Read the model definition and answer for the solid it produces. Units are mm, in the model's axes. Coordinates: 2 decimals unless noted, no trailing zeros. Write each loop counter-clockwise with the first axis right and the second up, starting at its lowest first coordinate (ties: lowest second). Pieces come first, ordered by that corner, then holes. Notation, with made-up numbers: (24.5, 86) -> (48.5, 86) arc R14 ccw to (48.5, 110) -> close; hole circle Ø8 at (4.5, 43). An arc over 180 degrees is marked (long way). Answer in a Markdown table with one row per item. Add a question column.
Item 1: Section C-C on y = 2.4 is taken. Count the separate pieces of the cut face and the enclosed holes in it, then the cut area to 3 significant figures.
Item 2: Given pin 1 Ø0.9 at (x, y) = (148, 2) entering from -Z; pin 2 Ø0.9 at (y, z) = (1, -73.5) entering from -X, each flat-ended and moving along its own axis, determine where each tip first touches the part or whether it passes through.
Item 3: Section A-A on z = -174 is taken. Write down the section's boundary in (x, y), then the cut area to 3 significant figures.
Item 4: Section B-B on z = -23 is taken. Write down the section's boundary in (x, y), then the cut area to 3 significant figures.
Item 5: Straight lines are drawn through the part: line 1 (X direction, y = 1.9, z = -97); line 2 (X direction, y = 1.95, z = -175.5); line 3 (Z direction, x = 139.2, y = 2). For each, find the intervals that lie inside material, in ascending order. Write a range as from..to.
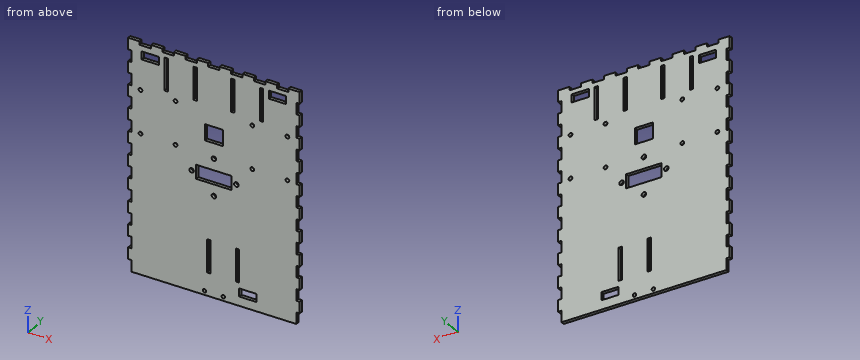
```python
from build123d import *

# Parameters (mm, degrees)
MDFESB_W          = 150
MDFESB_H          = 200
MDF_DEPTH         = 3
LDRESB_W          = 3
LDRESB_H          = 28.5
LDRESB_W_2        = 15
LDRESB_H_2        = 7
LDRBURACOS_DEPTH  = 3
CORESB_R          = 2
CORESB_W          = 31.12
CORESB_H          = 12.13
CORBURACOS_DEPTH  = 3
ENCAIXESESB_W     = 10
ENCAIXESESB_H     = 3
ENCAIXESESB_W_2   = 3
ENCAIXESESB_H_2   = 10
ENCAIXE_DEPTH     = 3
ACOPLMOTORESB_R   = 1.65
ACOPLMOTORESB_W   = 16
ACOPLMOTORESB_H   = 14
ACOPLMOTOR_DEPTH  = 3
CASTERFUROSESB_R  = 1.5
CASTERFUROS_DEPTH = 3


with BuildPart() as part:
    # mdfEsb → mdf (new body)
    with BuildSketch(Plane(origin=(0, 0, 0), x_dir=(1, 0, 0), z_dir=(0, 1, 0))):
        with Locations((75, 100)):
            Rectangle(MDFESB_W, MDFESB_H)
    extrude(amount=MDF_DEPTH)

    # ldrEsb → ldrBuracos (cut)
    with BuildSketch(Plane(origin=(0, 3, 0), x_dir=(1, 0, 0), z_dir=(0, 1, 0))):
        with Locations((33.4, 21.25)):
            Rectangle(LDRESB_W, LDRESB_H)
        with Locations((58.5, 21.25)):
            Rectangle(LDRESB_W, LDRESB_H)
        with Locations((91.5, 21.25)):
            Rectangle(LDRESB_W, LDRESB_H)
        with Locations((116.6, 21.25)):
            Rectangle(LDRESB_W, LDRESB_H)
        with Locations((70.5, 165.75)):
            Rectangle(LDRESB_W, LDRESB_H)
        with Locations((95.6, 165.75)):
            Rectangle(LDRESB_W, LDRESB_H)
        with Locations((130.6, 10.5)):
            Rectangle(LDRESB_W_2, LDRESB_H_2)
        with Locations((19.4, 11.5)):
            Rectangle(LDRESB_W_2, LDRESB_H_2)
        with Locations((104.6, 188.5)):
            Rectangle(LDRESB_W_2, LDRESB_H_2)
    extrude(amount=-LDRBURACOS_DEPTH, mode=Mode.SUBTRACT)

    # corEsb → corBuracos (cut)
    with BuildSketch(Plane(origin=(0, 3, 0), x_dir=(1, 0, 0), z_dir=(0, 1, 0))):
        with Locations(Location((75, 112.63, 0), (0, 0, 270))):
            Circle(CORESB_R)
        with Locations(Location((75, 80.5, 0), (0, 0, 270))):
            Circle(CORESB_R)
        with Locations(Location((94.56, 96.565, 0), (0, 0, 270))):
            Circle(CORESB_R)
        with Locations(Location((55.44, 96.565, 0), (0, 0, 270))):
            Circle(CORESB_R)
        with Locations((75, 96.565)):
            Rectangle(CORESB_W, CORESB_H)
    extrude(amount=-CORBURACOS_DEPTH, mode=Mode.SUBTRACT)

    # EncaixesEsb → Encaixe (cut)
    with BuildSketch(Plane(origin=(0, 3, 0), x_dir=(1, 0, 0), z_dir=(0, 1, 0))):
        with Locations((15, 1.5)):
            Rectangle(ENCAIXESESB_W, ENCAIXESESB_H)
        with Locations((1.5, 35)):
            Rectangle(ENCAIXESESB_W_2, ENCAIXESESB_H_2)
        with Locations((1.5, 15)):
            Rectangle(ENCAIXESESB_W_2, ENCAIXESESB_H_2)
        with Locations((1.5, 55)):
            Rectangle(ENCAIXESESB_W_2, ENCAIXESESB_H_2)
        with Locations((1.5, 75)):
            Rectangle(ENCAIXESESB_W_2, ENCAIXESESB_H_2)
        with Locations((1.5, 95)):
            Rectangle(ENCAIXESESB_W_2, ENCAIXESESB_H_2)
        with Locations((1.5, 115)):
            Rectangle(ENCAIXESESB_W_2, ENCAIXESESB_H_2)
        with Locations((1.5, 135)):
            Rectangle(ENCAIXESESB_W_2, ENCAIXESESB_H_2)
        with Locations((1.5, 155)):
            Rectangle(ENCAIXESESB_W_2, ENCAIXESESB_H_2)
        with Locations((1.5, 175)):
            Rectangle(ENCAIXESESB_W_2, ENCAIXESESB_H_2)
        with Locations((1.5, 195)):
            Rectangle(ENCAIXESESB_W_2, ENCAIXESESB_H_2)
        with Locations((35, 1.5)):
            Rectangle(ENCAIXESESB_W, ENCAIXESESB_H)
        with Locations((55, 1.5)):
            Rectangle(ENCAIXESESB_W, ENCAIXESESB_H)
        with Locations((75, 1.5)):
            Rectangle(ENCAIXESESB_W, ENCAIXESESB_H)
        with Locations((95, 1.5)):
            Rectangle(ENCAIXESESB_W, ENCAIXESESB_H)
        with Locations((115, 1.5)):
            Rectangle(ENCAIXESESB_W, ENCAIXESESB_H)
        with Locations((135, 1.5)):
            Rectangle(ENCAIXESESB_W, ENCAIXESESB_H)
        with Locations((148.5, 35)):
            Rectangle(ENCAIXESESB_W_2, ENCAIXESESB_H_2)
        with Locations((148.5, 15)):
            Rectangle(ENCAIXESESB_W_2, ENCAIXESESB_H_2)
        with Locations((148.5, 55)):
            Rectangle(ENCAIXESESB_W_2, ENCAIXESESB_H_2)
        with Locations((148.5, 75)):
            Rectangle(ENCAIXESESB_W_2, ENCAIXESESB_H_2)
        with Locations((148.5, 95)):
            Rectangle(ENCAIXESESB_W_2, ENCAIXESESB_H_2)
        with Locations((148.5, 115)):
            Rectangle(ENCAIXESESB_W_2, ENCAIXESESB_H_2)
        with Locations((148.5, 135)):
            Rectangle(ENCAIXESESB_W_2, ENCAIXESESB_H_2)
        with Locations((148.5, 155)):
            Rectangle(ENCAIXESESB_W_2, ENCAIXESESB_H_2)
        with Locations((148.5, 175)):
            Rectangle(ENCAIXESESB_W_2, ENCAIXESESB_H_2)
        with Locations((148.5, 195)):
            Rectangle(ENCAIXESESB_W_2, ENCAIXESESB_H_2)
    extrude(amount=-ENCAIXE_DEPTH, mode=Mode.SUBTRACT)

    # AcoplMotorEsb → AcoplMotor (cut)
    with BuildSketch(Plane(origin=(0, 3, 0), x_dir=(1, 0, 0), z_dir=(0, 1, 0))):
        with Locations(Location((108.56, 41.5, 0), (0, 0, 270))):
            Circle(ACOPLMOTORESB_R)
        with Locations(Location((108.56, 79, 0), (0, 0, 270))):
            Circle(ACOPLMOTORESB_R)
        with Locations(Location((139.2, 41.5, 0), (0, 0, 270))):
            Circle(ACOPLMOTORESB_R)
        with Locations(Location((139.2, 79, 0), (0, 0, 270))):
            Circle(ACOPLMOTORESB_R)
        with Locations(Location((10.8, 79, 0), (0, 0, 90))):
            Circle(ACOPLMOTORESB_R)
        with Locations(Location((10.8, 41.5, 0), (0, 0, 90))):
            Circle(ACOPLMOTORESB_R)
        with Locations(Location((41.44, 79, 0), (0, 0, 90))):
            Circle(ACOPLMOTORESB_R)
        with Locations(Location((41.44, 41.5, 0), (0, 0, 90))):
            Circle(ACOPLMOTORESB_R)
        with Locations((75, 60.25)):
            Rectangle(ACOPLMOTORESB_W, ACOPLMOTORESB_H)
    extrude(amount=-ACOPLMOTOR_DEPTH, mode=Mode.SUBTRACT)

    # CasterFurosEsb → CasterFuros (cut)
    with BuildSketch(Plane(origin=(0, 3, 0), x_dir=(1, 0, 0), z_dir=(0, 1, 0))):
        with Locations(Location((66.75, 196.5, 0), (0, 0, 270))):
            Circle(CASTERFUROSESB_R)
        with Locations(Location((83.25, 196.5, 0), (0, 0, 90))):
            Circle(CASTERFUROSESB_R)
    extrude(amount=-CASTERFUROS_DEPTH, mode=Mode.SUBTRACT)


solid = part.part
```
Results below:
| question | item | result |
|---|---|---|
| 1 | separate pieces | 1 |
| 1 | enclosed holes | 25 |
| 1 | area | 27,600 mm2 |
| 2 | pin 1 | stops at z = -190 |
| 2 | pin 2 | stops at x = 3 |
| 3 | outline | (3, 0) -> (69, 0) -> (69, 3) -> (3, 3) -> close; (72, 0) -> (94.1, 0) -> (94.1, 3) -> (72, 3) -> close; (97.1, 0) -> (147, 0) -> (147, 3) -> (97.1, 3) -> close |
| 3 | area | 414 mm2 |
| 4 | outline | (0, 0) -> (31.9, 0) -> (31.9, 3) -> (0, 3) -> close; (34.9, 0) -> (57, 0) -> (57, 3) -> (34.9, 3) -> close; (60, 0) -> (90, 0) -> (90, 3) -> (60, 3) -> close; (93, 0) -> (115.1, 0) -> (115.1, 3) -> (93, 3) -> close; (118.1, 0) -> (150, 0) -> (150, 3) -> (118.1, 3) -> close |
| 4 | area | 414 mm2 |
| 5 | line 1 | x = 3..53.49, 57.39..59.44, 90.56..92.61, 96.51..147 |
| 5 | line 2 | x = 3..69, 72..94.1, 97.1..147 |
| 5 | line 3 | z = -200..-80.65, -77.35..-43.15, -39.85..-3 |
